Model file for the job. Use its own axes, mm. A direction names the side the tool comes from. Round coordinates to 2 decimals unless told otherwise and drop trailing zeros. Order: outer loops, then holes, each group sorted by start corner. A loop starts at its lowest first (then second) coordinate and runs counter-clockwise, first axis right, second up. Notation, with made-up numbers: M 36,64.25 L 80,64.25 A32 ccw 80,95.25 Z; hole C -17.5,34 d8. An arc over 180 degrees is marked long. Return JSON: item names as keys, results as strings. Group by question number.
Item 1: Pin check, flat tips, straight feed: pin 1 Ø1 at (x, z) = (15, 0) entering from +Y; pin 2 Ø0.5 at (x, z) = (17.5, 0) entering from +Y. Stop position of each tip, or through.
Item 2: Slice it at B-B on x = 23.75. Write the cut outline in (y, z).
Item 3: Probe line 1 along Z through (x, y) = (18.5, -7.5); line 2 along Y through (x, z) = (23.75, 0.1). List the from-to ranges inside material, lowest first.
Item 4: Slice it at A-A on y = -7.5. Write the cut outline in (x, z), then the cut area to 3 significant figures.
Item 5: Pull direction Z, two halves, no side cores. Call faces 4 (the face through (15, 0, -2.5)), 5 (the face through (15, -8, 0.3)), 6 (the face through (15, 10, -1)), 7 (the face through (15, 8, -0.3)): pulls with the +Z half, pulls with the -Z half, needs draft (parallel to the pull), parting line crosses it, or undercut.
Item 6: Which spindle directions (+Z, -Z, +X, -X, +Y, -Y) get a long thin tool onto all of the face, cutting with end or side? Do faces 1 (the face through (15, 0, 2.5)), 2 (the face through (15, 8, 0.3)), 3 (the face through (15, -8, -0.3)). Say none if no direction does.
from build123d import *

# Parameters (mm, degrees)
SKETCH4_W           = 5
SKETCH4_H           = 20
BOSS_EXTRUDE2_DEPTH = 30
CUT_EXTRUDE3_DEPTH  = 31


with BuildPart() as part:
    # Sketch4 → Boss-Extrude2 (new body)
    with BuildSketch(Plane(origin=(0, 0, 0), x_dir=(0, 0, -1), z_dir=(1, 0, 0))):
        Rectangle(SKETCH4_W, SKETCH4_H)
    extrude(amount=BOSS_EXTRUDE2_DEPTH)

    # Sketch5 → Cut-Extrude3 (cut, through all)
    with BuildSketch(Plane(origin=(30, 0, 0), x_dir=(0, 0, -1), z_dir=(1, 0, 0))):
        Polygon((0.3, 6.8), (0.3, 10), (0, 10), (-0.3, 10), (-0.3, 6.8), align=None)
    cut_extrude3 = extrude(amount=-CUT_EXTRUDE3_DEPTH, mode=Mode.SUBTRACT)

    # Mirror3: Cut-Extrude3 across plane
    add(cut_extrude3.mirror(Plane.ZX), mode=Mode.SUBTRACT)


solid = part.part
Output values:
{
 "1": {"pin 1": "y = 10", "pin 2": "y = 6.8"},
 "2": {"outline": "M -10,-2.5 L 10,-2.5 L 10,-0.3 L 6.8,-0.3 L 6.8,0.3 L 10,0.3 L 10,2.5 L -10,2.5 L -10,0.3 L -6.8,0.3 L -6.8,-0.3 L -10,-0.3 Z"},
 "3": {"line 1": "-2.5 to -0.3, 0.3 to 2.5", "line 2": "-6.8 to 6.8"},
 "4": {"outline": "M 0,-2.5 L 30,-2.5 L 30,-0.3 L 0,-0.3 Z; M 0,0.3 L 30,0.3 L 30,2.5 L 0,2.5 Z", "area": "132 mm²"},
 "5": {"face 4": "pulls with the -Z half", "face 5": "undercut", "face 6": "needs draft", "face 7": "undercut"},
 "6": {"face 1": "+Z, +X, -X, +Y, -Y", "face 2": "+X, -X, +Y", "face 3": "+X, -X, -Y"}
}
